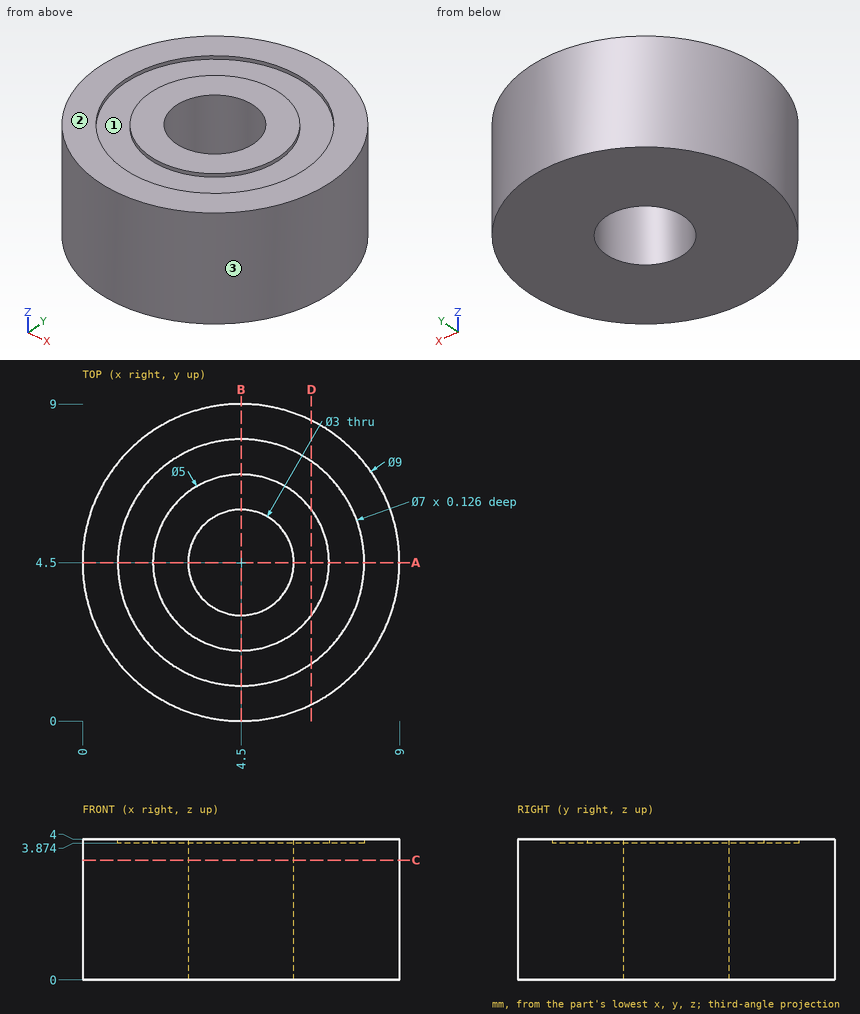
Geometry: see drawing. Coordinates: mm, zero at the bounding-box minimum. Round coordinates to 2 decimals unless told otherwise and drop trailing zeros. Loops run counter-clockwise (first coordinate to the right, second up) from the corner with the lowest first, then second, coordinate; pieces in that order, holes last. Notation, with made-up numbers: (18, 11) -> (57, 11) arc R29 ccw to (57, 49) -> close; hole circle Ø3 at (-15, 15). An arc over 180 degrees is marked (long way). Use one line per item in the form item = value. Start each with the question number.
Item 1: Mould query, pull axis X, two halves, no side actions, for the marked faces 1, 2 and 3. Classes: pulls with the +X half, pulls with the -X half, needs draft (parallel to the pull), parting line crosses it, or undercut.
Item 2: Section query C-C on z = 3.4. Return the cut outline in (x, y).
Item 3: Section query D-D on x = 6.5. Return the cut outline in (y, z).
Item 4: Material intervals for L1, parallel to X at y = 4.25, z = 3.2; L2, parallel to Y at x = 4.5, z = 1; L3, parallel to X at y = 4, z = 3 (1 decimal), sorted ascending. Write a range as from..to.
Item 5: Section query A-A on y = 4.5. Return the cut outline in (x, z).
Ans:
q1.face_1 = undercut
q1.face_2 = needs draft
q1.face_3 = parting line crosses it
q2.outline = circle Ø9 at (4.5, 4.5); hole circle Ø3 at (4.5, 4.5)
q3.outline = (0.47, 0) -> (8.53, 0) -> (8.53, 4) -> (7.37, 4) -> (7.37, 3.87) -> (6, 3.87) -> (6, 4) -> (3, 4) -> (3, 3.87) -> (1.63, 3.87) -> (1.63, 4) -> (0.47, 4) -> close
q4.L1 = 0.01..3.02, 5.98..8.99
q4.L2 = 0..3, 6..9
q4.L3 = 0..3.1, 5.9..9
q5.outline = (0, 0) -> (3, 0) -> (3, 4) -> (2, 4) -> (2, 3.87) -> (1, 3.87) -> (1, 4) -> (0, 4) -> close; (6, 0) -> (9, 0) -> (9, 4) -> (8, 4) -> (8, 3.87) -> (7, 3.87) -> (7, 4) -> (6, 4) -> close
